Part print with two shaded views. Sizes in mm from the minimum x, y, z corner. A direction names the side the tool comes from. Coordinates: 2 decimals unless noted, no trailing zeros. Order: outer loops, then holes, each group sorted by start corner. A loop starts at its lowest first (then second) coordinate and runs counter-clockwise, first axis right, second up.
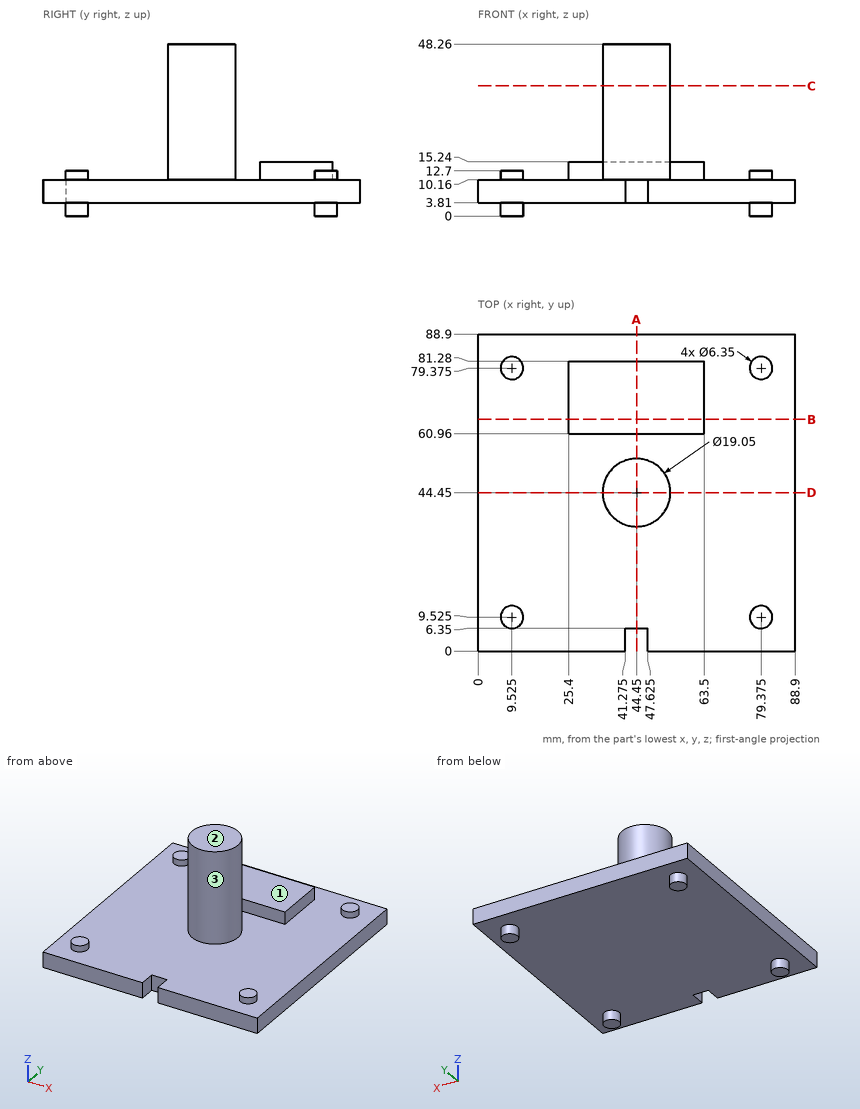
Q1. Which spindle directions (+Z, -Z, +X, -X, +Y, -Y) get a long thin tool onto all of the face, cutting with end or side? Do the marked faces 1, 2 and 3. Say none if no direction does.
Results list:
face 1: +Z, +X, -X, +Y
face 2: +Z, +X, -X, +Y, -Y
face 3: +Z
Q2. Cut at A-A on x = 44.45. Write the cut outline in (y, z) (3 decimals), and give its area (3 significant figures).
Results list:
outline: (6.35, 3.81) - (88.9, 3.81) - (88.9, 10.16) - (81.28, 10.16) - (81.28, 15.24) - (60.96, 15.24) - (60.96, 10.16) - (53.975, 10.16) - (53.975, 48.26) - (34.925, 48.26) - (34.925, 10.16) - (6.35, 10.16) - close
area: 1,350 mm2
Q3. Pin check, flat tips, straight feed: pin 1 Ø3 at (x, z) = (52, 27) entering from +Y; pin 2 Ø22.5 at (x, y) = (53.5, 67) entering from +Z; pin 3 Ø2.5 at (x, z) = (42.5, 11.5) entering from -Y; pin 4 Ø7 at (y, z) = (4.5, 7) entering from -X. Stop position of each tip, or through.
Results list:
pin 1: stops at y = 51.81
pin 2: stops at z = 15.24
pin 3: stops at y = 34.95
pin 4: stops at x = 0
Q4. Cut at B-B on y = 65. Write the cut outline in (x, z).
Results list:
outline: (0, 3.81) - (88.9, 3.81) - (88.9, 10.16) - (63.5, 10.16) - (63.5, 15.24) - (25.4, 15.24) - (25.4, 10.16) - (0, 10.16) - close
Q5. Cut at D-D on y = 44.45. Write the cut outline in (x, z) (3 decimals), and give its area (3 significant figures).
Results list:
outline: (0, 3.81) - (88.9, 3.81) - (88.9, 10.16) - (53.975, 10.16) - (53.975, 48.26) - (34.925, 48.26) - (34.925, 10.16) - (0, 10.16) - close
area: 1,290 mm2
Q6. Cut at C-C on z = 36.5. Write the cut outline in (x, y) (3 decimals).
Results list:
outline: circle Ø19.05 at (44.45, 44.45)
Q7. Wall check: line 1 along Z through (x, y) = (4, 37); line 2 along Y through (x, z) = (60.5, 13.5); line 3 along Z through (x, y) = (11, 80). Give the ranges that are in metal, low to high.
Results list:
line 1: z = 3.81 to 10.16
line 2: y = 60.96 to 81.28
line 3: z = 0 to 12.7
